Autodesk Inventor part; units mm, degrees
ref_plane "YZ Plane" through (0, 0, 0) normal (1, 0, 0) x (0, 1, 0)
ref_plane "XZ Plane" through (0, 0, 0) normal (0, 1, 0) x (-1, 0, 0)
ref_plane "XY Plane" through (0, 0, 0) normal (0, 0, 1) x (1, 0, 0)
sketch "Sketch1" plane through (0, 0, 0) normal (0, 1, 0) x (-1, 0, 0)
  line L0 (-7.9375, 23.8125) -> (7.9375, 23.8125)
  line L1 (11.1125, 20.6375) -> (11.1125, -20.6375)
  line L2 (7.9375, -23.8125) -> (-7.9375, -23.8125)
  line L3 (-11.1125, -20.6375) -> (-11.1125, 20.6375)
  line L4 (-11.1125, 23.8125) -> (11.1125, -23.8125) construction
  line L5 (11.1125, 23.8125) -> (-11.1125, -23.8125) construction
  arc A0 (7.9375, -23.8125) -> (11.1125, -20.6375) centre (7.9375, -20.6375) ccw
  arc A1 (-11.1125, -20.6375) -> (-7.9375, -23.8125) centre (-7.9375, -20.6375) ccw
  arc A2 (-7.9375, 23.8125) -> (-11.1125, 20.6375) centre (-7.9375, 20.6375) ccw
  arc A3 (11.1125, 20.6375) -> (7.9375, 23.8125) centre (7.9375, 20.6375) ccw
  point P0 (0, 0)
  dimension "d0" = 47.625
  dimension "d1" = 22.225
  dimension "d15" = 3.175
extrude "Extrusion1" add sketch "Sketch1" along normal mid plane 12.065
sketch "Sketch3" plane through (0, -6.0325, -23.8125) normal (1, 0, 0) x (0, 0, -1)
  line L0 (-44.45, 12.065) -> (-3.175, 12.065)
  line L1 (-3.175, 0) -> (-44.45, 0)
  line L2 (-49.2125, 12.065) -> (1.5875, 12.065)
  arc A0 (-47.625, 13.6525) -> (-49.2125, 12.065) centre (-47.2211, 11.6611) ccw
  arc A1 (1.5875, 12.065) -> (0, 13.6525) centre (-0.4039, 11.6611) ccw
  arc A2 (0, 13.6525) -> (-47.625, 13.6525) centre (-23.8125, -103.7429) ccw
  line L3 (-3.175, 12.065) -> (-3.175, 0)
  line L4 (-44.45, 12.065) -> (-44.45, 0)
  point P0 (-23.8125, 6.0325)
  point P1 (-47.625, 12.065)
  dimension "d5" = 50.8
  dimension "d9" = 1.5875
  dimension "d13" = 2.032
  dimension "d14" = 2.032
extrude "Extrusion2" add sketch "Sketch3" along normal mid plane 25.4 contours L2 A0 A2 A1 L0
fillet "Fillet1" radius 1.27 6 edges at (-12.7, 7.0654, -24.8454) (-12.7, 7.0654, 24.8454) (-12.7, 10.0107, 0) (12.7, 7.0654, 24.8454) (12.7, 7.0654, -24.8454) (12.7, 10.0107, 0)
properties part number "ARM_029_BottomIntakeSide_Cap" material "ABS Plastic"
Here's how the part is built. I have some questions about the finished solid (model axes, mm). A direction names the side the tool comes from. Round coordinates to 2 decimals unless told otherwise and drop trailing zeros. Order: outer loops, then holes, each group sorted by start corner. A loop starts at its lowest first (then second) coordinate and runs counter-clockwise, first axis right, second up. Notation, with made-up numbers: M -8,-18.75 L 41,-18.75 A15 ccw 41,8.25 Z; hole C 75,26 d11. An arc over 180 degrees is marked long. Return JSON: item names as keys, results as strings. Group by question number.
1. Please list where these lines run through material, in increasing order: probe 1 along X at (y, z) = (5, -20); probe 2 along Z at (x, y) = (7.5, 2.25); probe 3 along Z at (x, y) = (10, 7).
2. On a 3-axis mill with a long thin cutter (end or side, diameter ignored), from which of +Z, -Z, +X, -X, +Y, -Y can I reach the whole of each face in a straight line? I mean faces 1 (the face through (11.112, 0, 0)), 2 (the face through (-10.207, -0.084, -22.858)), 3 (the face through (10.158, -0.084, -22.907)), 4 (the face through (-11.3, 6.032, 2)), 5 (the face through (0, 0, 23.812)). Say none if no direction works.
3. If we section it at A-A on x = 1.5: List the corners of the cut face in (y, z) for me.
4. I'm going to push flat-ended pins straight in: pin 1 Ø1 at (x, y) = (-1.5, -3.5) entering from +Z; pin 2 Ø1 at (x, z) = (-2.5, -6.5) entering from +Y; pin 3 Ø3 at (x, y) = (9.5, 1) entering from -Z. Where does each tip first touch, or does it pass through?
Reply:
{
 "1": {"probe 1": "-11.11 to 11.11", "probe 2": "-23.81 to 23.81", "probe 3": "-24.91 to 24.91"},
 "2": {"face 1": "+Z, -Z, +X, -Y", "face 2": "-Z, -X, -Y", "face 3": "-Z, +X, -Y", "face 4": "-Y", "face 5": "+Z, +X, -X, -Y"},
 "3": {"outline": "M -6.03,-23.81 L 6.03,-23.81 L 6.03,-25.4 A2.03 ccw 7.62,-23.81 A119.79 ccw 7.62,23.81 A2.03 ccw 6.03,25.4 L 6.03,23.81 L -6.03,23.81 Z"},
 "4": {"pin 1": "z = 23.81", "pin 2": "y = 9.86", "pin 3": "z = -23.81"}
}
